Build history of the part. All positions in model axes, mm. Give positions to 0.01 mm unless a question says otherwise; leave off trailing zeros. Order: outer loops, then holes, each group sorted by start corner. A loop starts at its lowest first (then second) coordinate and runs counter-clockwise, first axis right, second up. Notation, with made-up numbers: M 15,27 L 29,27 A19 cw 29,47 Z; hole C 55.25,8.5 d2. An arc over 180 degrees is marked long. Use CSV: the item, a comma, the result in double quotes. Start each with the question number.
Item 1: Band-saw the part on B-B on x = 5.5. Write the cut outline in (y, z).
Item 2: Band-saw the part on D-D on z = 0.5. Write the cut outline in (x, y), plus the area to 3 significant figures.
Item 3: Wall check: line 1 along Y through (x, z) = (5.5, 1.4); line 2 along Y through (x, z) = (4.5, 1.6); line 3 along X through (y, z) = (70.5, 0.55). Give the ranges that are in metal, low to high.
Item 4: Pin check, flat tips, straight feed: P1, Ø2, axis at x = -2.7, y = 50, coming from the -Z side; P2, Ø1, axis at y = 52, z = 1, coming from the +X side. Stop position of each tip, or through.
Item 5: Band-saw the part on A-A on y = 50. Write the cut outline in (x, z), plus the area to 3 significant figures.
Item 6: Band-saw the part on C-C on x = -2.25. Write the cut outline in (y, z).
from build123d import *

# Parameters (mm, degrees)
SKETCH_1_R          = 1.65
EXTRUDE_1_DEPTH     = 2
SKETCH_2_OUTSIDE_W  = 35.044
SKETCH_2_OUTSIDE_H  = 96.312
SKETCH_2_OUTSIDE_R  = 32.015621187
CUT_EXTRUDE_1_DEPTH = 10


with BuildPart() as part:
    # 草图1 → 凸台-拉伸1 (new body)
    with BuildSketch(Plane.XY):
        with BuildLine():
            Line((10, 68.284271247), (10, 78.284271247))
            ThreePointArc((10, 78.284271247), (-6.350322366, 56.492864354), (0, 30))
            Line((0, 30), (0, 0))
            Line((0, 0), (10, 0))
            Line((10, 0), (10, 31.715728753))
            ThreePointArc((10, 31.715728753), (1.350167547, 50), (10, 68.284271247))
        make_face()
        with Locations((5, 5)):
            Circle(SKETCH_1_R, mode=Mode.SUBTRACT)
        with Locations((5, 17)):
            Circle(SKETCH_1_R, mode=Mode.SUBTRACT)
        with Locations((-2.697604364, 50)):
            Circle(SKETCH_1_R, mode=Mode.SUBTRACT)
        with Locations((5, 69.161348792)):
            Circle(SKETCH_1_R, mode=Mode.SUBTRACT)
        with Locations((5, 30.838651208)):
            Circle(SKETCH_1_R, mode=Mode.SUBTRACT)
    extrude(amount=EXTRUDE_1_DEPTH)

    # 草图2 outside → 切除-拉伸1 (cut)
    with BuildSketch(Plane.XY.offset(2)):
        with Locations((1.492, 39.142)):
            Rectangle(SKETCH_2_OUTSIDE_W, SKETCH_2_OUTSIDE_H)
        with Locations((25, 50)):
            Circle(SKETCH_2_OUTSIDE_R, mode=Mode.SUBTRACT)
    extrude(amount=-CUT_EXTRUDE_1_DEPTH, mode=Mode.SUBTRACT)


solid = part.part
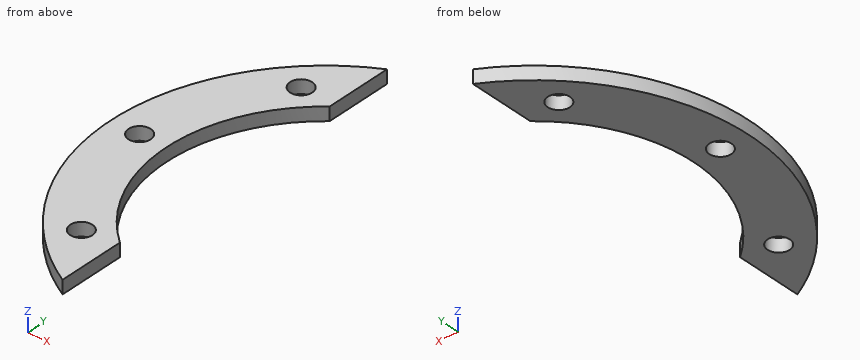
Model answer:
1,outline,"M 24.61,0 L 29.27,0 L 29.27,2 L 24.61,2 Z; M 32.41,0 L 36.62,0 L 36.62,2 L 32.41,2 Z; M 63.38,0 L 67.59,0 L 67.59,2 L 63.38,2 Z; M 70.73,0 L 75.39,0 L 75.39,2 L 70.73,2 Z"
2,outline,"M 10,21.72 L 10,31.72 A23.65 cw 10,68.28 L 10,78.28 A32.02 ccw Z; hole C -2.7,50 d3.3; hole C 5,30.84 d3.3; hole C 5,69.16 d3.3"
2,area,"440 mm^2"
3,line 1,"y = 24.61 to 29.27, 32.41 to 36.62, 63.38 to 67.59, 70.73 to 75.39"
3,line 2,"y = 25.41 to 29.27, 32.41 to 38.21, 61.79 to 67.59, 70.73 to 74.59"
3,line 3,"x = 0.41 to 4.04, 5.96 to 10"
4,P1,"passes through"
4,P2,"stops at x = 1.48"
5,outline,"M -7.02,0 L -4.35,0 L -4.35,2 L -7.02,2 Z; M -1.05,0 L 1.35,0 L 1.35,2 L -1.05,2 Z"
5,area,"10.1 mm^2"
6,outline,"M 33.19,0 L 48.41,0 L 48.41,2 L 33.19,2 Z; M 51.59,0 L 66.81,0 L 66.81,2 L 51.59,2 Z"
